Check sheet for the modelled part. Datum: model origin and axes. Units: mm. Face numbers are marked on the shaded views. Give positions to 0.01 mm unless a question says otherwise; leave off trailing zeros. Write each loop counter-clockwise with the first axis right and the second up, starting at its lowest first coordinate (ties: lowest second). Pieces come first, ordered by that corner, then holes. Notation, with made-up numbers: (-8.5, 78) -> (7.5, 78) arc R16 ccw to (7.5, 90) -> close; hole circle Ø2 at (23.5, 64.25). An arc over 180 degrees is marked (long way). Use a Markdown table: item, result. Add a question column.
1. Scan lines: probe 1 along Y at (x, z) = (0, 44); probe 2 along Z at (x, y) = (6, 10); probe 3 along X at (y, z) = (-1, 48). Record each from-to range of solid material in increasing order. Write a range as [from, to].
2. Gauge pin test, flat ends, axial feed: P1, Ø12, axis at x = 19.5, z = 7.5, coming from the -Y side; P2, Ø12, axis at y = 17, z = 42, coming from the +X side; P3, Ø5, axis at x = 12.5, z = 30.5, coming from the -Y side. Record the tip position at first contact, or that the pin passes through.
3. Cross-section at A-A (x = 0). Enter the section's corners in (y, z), then the cut area to 3 significant figures.
4. Release check for a two-part mould opening along Y. For the marked faces 1, 2 and 3 record: released by +Y, released by -Y, zero draft, split by the parting line, or undercut.
5. Cross-section at C-C (z = 46.5). Enter the section's corners in (x, y), then the cut area to 3 significant figures.
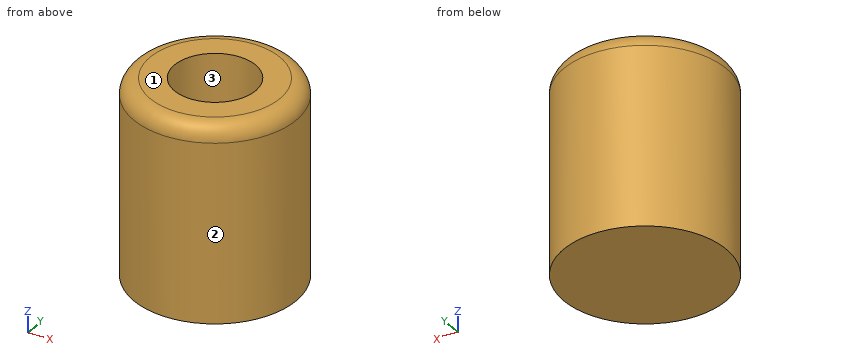
from build123d import *

# Parameters (mm, degrees)
F0_R     = 12.5
F1_DEPTH = 25
F0_R_2   = 25
F2_DEPTH = 60
F3_R     = 5


with BuildPart() as f1:
    # F0 (on Top) → F1 (new body)
    with BuildSketch(Plane.XY):
        Circle(F0_R)
    extrude(amount=F1_DEPTH)

    # F0 (on Top) → F2 (join)
    with BuildSketch(Plane.XY):
        Circle(F0_R_2)
        Circle(F0_R, mode=Mode.SUBTRACT)
    extrude(amount=F2_DEPTH)

    # F3
    f3_edges = [f1.edges().sort_by_distance(p)[0] for p in [
        (-25, 0, 60),
    ]]
    fillet(f3_edges, radius=F3_R)


solid = f1.part
Worked answers:
| question | item | result |
|---|---|---|
| 1 | probe 1 | y = [-25, -12.5], [12.5, 25] |
| 1 | probe 2 | z = [0, 25] |
| 1 | probe 3 | x = [-24.98, -12.46], [12.46, 24.98] |
| 2 | P1 | stops at y = -21.04 |
| 2 | P2 | stops at x = 22.45 |
| 2 | P3 | stops at y = -22.91 |
| 3 | outline | (-25, 0) -> (25, 0) -> (25, 55) arc R5 ccw to (20, 60) -> (12.5, 60) -> (12.5, 25) -> (-12.5, 25) -> (-12.5, 60) -> (-20, 60) arc R5 ccw to (-25, 55) -> close |
| 3 | area | 2,110 mm² |
| 4 | face 1 | zero draft |
| 4 | face 2 | split by the parting line |
| 4 | face 3 | undercut |
| 5 | outline | circle Ø50 at (0, 0); hole circle Ø25 at (0, 0) |
| 5 | area | 1,470 mm² |
